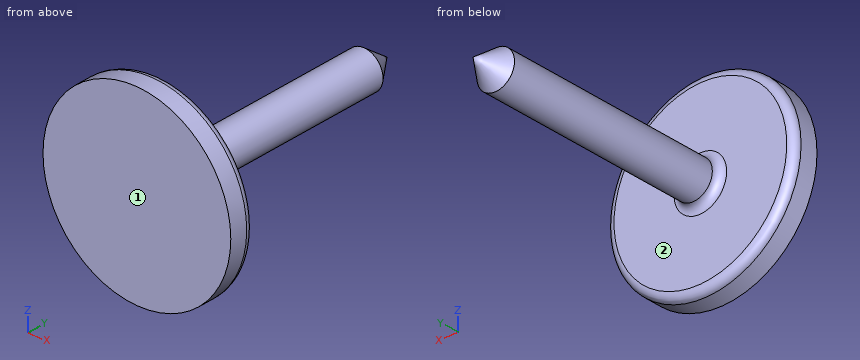
from build123d import *

# Parameters (mm, degrees)
RADYUS1_R = 3


with BuildPart() as part:
    # Çizim1 → Döndür1 (revolve)
    with BuildSketch(Plane.XY, mode=Mode.PRIVATE) as d_nd_r1_sk:
        Polygon((0, 0), (37.5, 0), (37.5, 10), (7.5, 10), (7.5, 100), (0, 110), align=None)
    revolve(d_nd_r1_sk.sketch.rotate(Axis((0, 0, 0), (0, 1, 0)), 90), axis=Axis((0, 0, 0), (0, 1, 0)))

    # Radyus1
    radyus1_edges = [part.edges().sort_by_distance(p)[0] for p in [
        (0, 10, 7.5),
        (0, 10, 37.5),
    ]]
    fillet(radyus1_edges, radius=RADYUS1_R)


solid = part.part
Could you check a few things on this model? Use its own coordinates, in mm. Face numbers are marked on the shaded views. A direction names the side the tool comes from. Round coordinates to 2 decimals unless told otherwise and drop trailing zeros. Loops run counter-clockwise (first coordinate to the right, second up) from the corner with the lowest first, then second, coordinate; pieces in that order, holes last. Notation, with made-up numbers: (-39.5, -6) - (10.5, -6) arc R6 cw to (10.5, 2) - close; hole circle Ø4 at (-26, 0.25). An arc over 180 degrees is marked (long way). Write item = value, one per line.
1) I'm going to push flat-ended pins straight in: P1, Ø5, axis at x = 28.5, z = 27.5, coming from the +Y side; P2, Ø8, axis at x = -0.5, y = 86, coming from the -Z side; P3, Ø3, axis at y = 33, z = -1.5, coming from the -X side. Where does each tip first touch, or does it pass through?
Computed:
P1 = 8.49
P2 = -7.5
P3 = -7.5
2) On a 3-axis mill with a long thin cutter (end or side, diameter ignored), from which of +Z, -Z, +X, -X, +Y, -Y can I reach the whole of each face in a straight line? I mean the marked faces 1 and 2. Say none if no direction works.
Computed:
face_1 = +Z, -Z, +X, -X, -Y
face_2 = +Y
3) Imagine slicing it at A-A (y = 66). Please give me the cut outline in (x, z).
Computed:
outline = circle Ø15 at (0, 0)
4) I need wall thicknesses on line 1 along Y through (x, z) = (19.5, -11.5); line 2 along Z through (x, y) = (23, 7); line 3 along Y through (x, z) = (0, -0.5). Which ranges of each line are inside material? Lowest first, please. Write a range as from..to.
Computed:
line_1 = 0..10
line_2 = -29.62..29.62
line_3 = 0..109.33
